Study the drawing (mm; zero at the part's minimum x, y, z) and answer. Give positions to 0.01 mm unless a question says otherwise; leave off trailing zeros. Order: outer loops, then holes, each group sorted by start corner. A loop starts at its lowest first (then second) coordinate and runs counter-clockwise, first axis right, second up.
Item 1: A cutting plane is placed at C-C (z = 32.5). Write down the section's boundary in (x, y) (1 decimal).
Item 2: A cutting plane is placed at B-B (x = 31). Write down the section's boundary in (y, z), plus the area to 3 significant figures.
Item 3: A cutting plane is placed at D-D (y = 32.5). Write down the section's boundary in (x, z).
Item 4: Given pin 1 Ø5 at (x, y) = (36, 21.5) entering from -Z; pin 2 Ø2 at (x, y) = (9, 37) entering from +Z, each flat-ended and moving along its own axis, determine where each tip first touches the part or whether it passes through.
Item 5: A cutting plane is placed at A-A (y = 16). Write down the section's boundary in (x, z) (1 decimal).
Item 6: The mould has two halves that part along X. Classify the marked faces 1, 2 and 3: +X half, -X half, draft (parallel to the pull), parting line (faces both ways), or undercut.
Item 7: Find the intervals of material crossed by line 1 along Z through (x, y) = (3, 20); line 2 along Z through (x, y) = (36, 24.5), in increasing order.
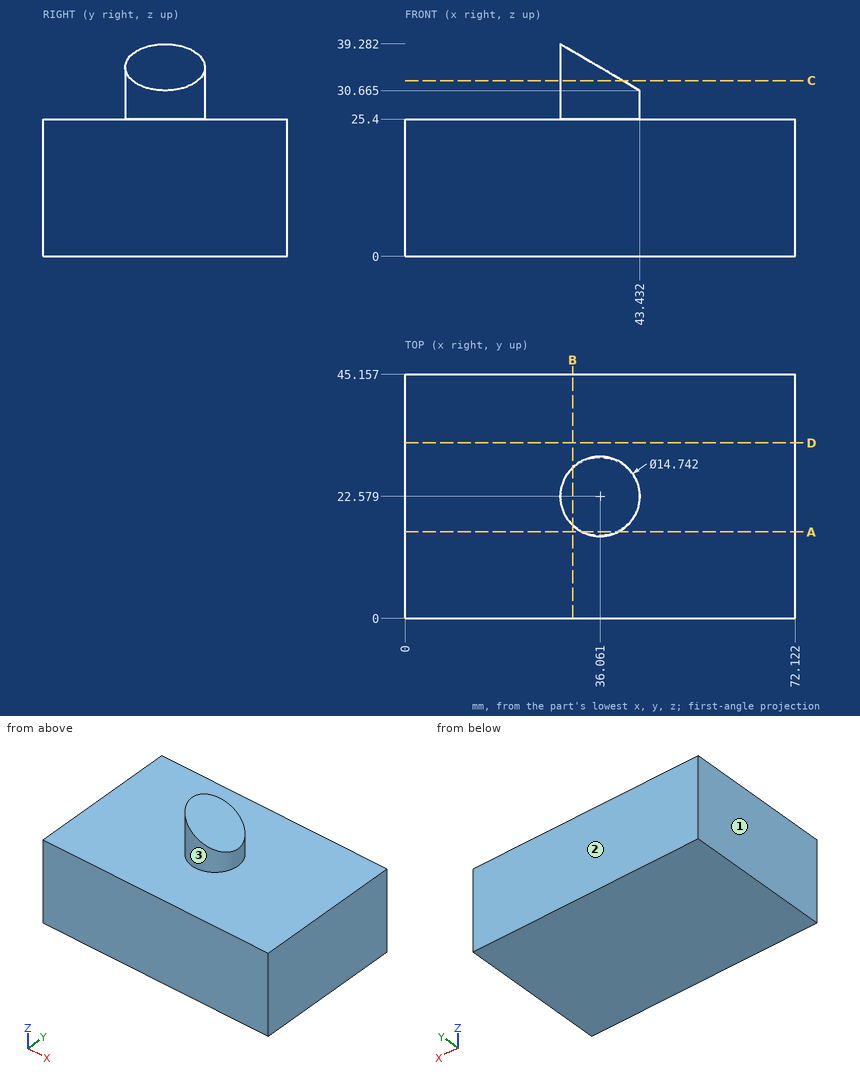
Response values:
1. outline: (40.3, 16.5) - (40.3, 28.6) arc R7.4 ccw (long way) to start
2. outline: (0, 0) - (45.16, 0) - (45.16, 25.4) - (27.94, 25.4) - (27.94, 37.93) - (17.22, 37.93) - (17.22, 25.4) - (0, 25.4) - close
2. area: 1,280 mm2
3. outline: (0, 0) - (72.12, 0) - (72.12, 25.4) - (0, 25.4) - close
4. pin 1: stops at z = 0
4. pin 2: stops at z = 25.4
5. outline: (0, 0) - (72.1, 0) - (72.1, 25.4) - (39.4, 25.4) - (39.4, 33) - (32.7, 36.9) - (32.7, 25.4) - (0, 25.4) - close
6. face 1: -X half
6. face 2: draft
6. face 3: parting line
7. line 1: z = 0 to 25.4
7. line 2: z = 0 to 35.01
